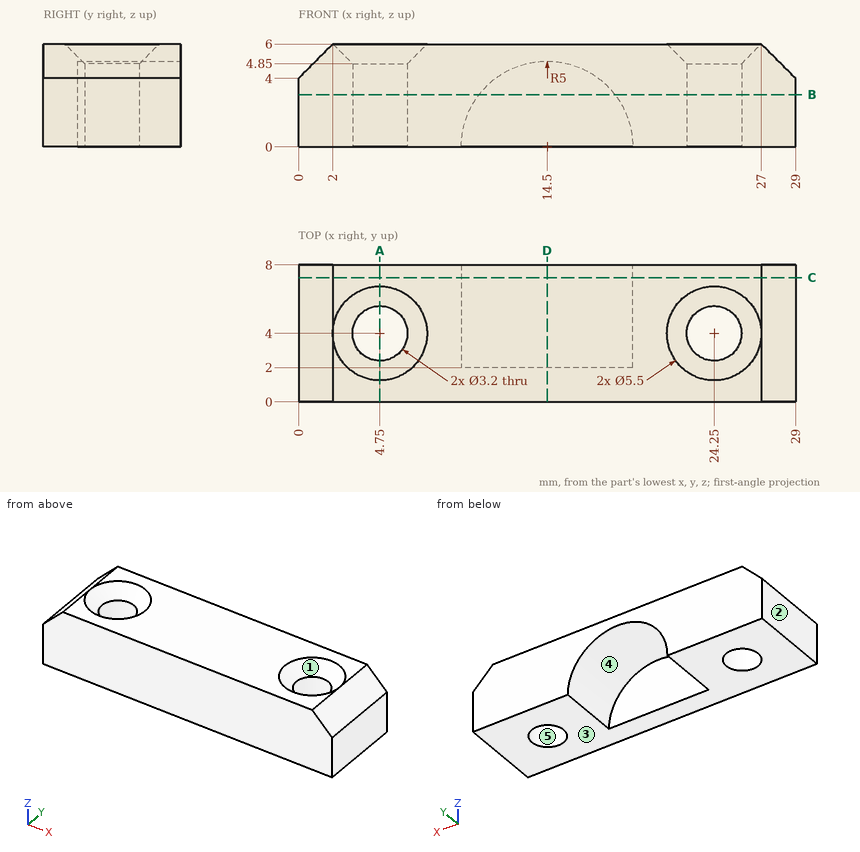
Here's the drawing with two shaded views (mm, measured from the low corner). I have some questions. A direction names the side the tool comes from. Coordinates: 2 decimals unless noted, no trailing zeros. Order: outer loops, then holes, each group sorted by start corner. A loop starts at its lowest first (then second) coordinate and runs counter-clockwise, first axis right, second up.
Item 1: For P1, Ø1.5, axis at x = 16, z = 3, coming from the +Y side; P2, Ø1.5, axis at y = 3, z = 5, coming from the -X side, each with a flat end and sliding along its axis, tell me the tip position at first contact or that it passes through.
Result sheet:
P1: stops at y = 2
P2: stops at x = 0.25
Item 2: If we section it at C-C on y = 7.25: List the corners of the cut face in (x, z) for me.
Result sheet:
outline: (0, 0) - (9.5, 0) arc R5 cw to (19.5, 0) - (29, 0) - (29, 4) - (27, 6) - (2, 6) - (0, 4) - close
Item 3: I need wall thicknesses on line 1 (Y direction, x = 24.25, z = 2.5); line 2 (X direction, y = 3.25, z = 2.9); line 3 (X direction, y = 4.25, z = 5.45). Which ranges of each line are inside material? Lowest first, please.
Result sheet:
line 1: y = 0 to 2.4, 5.6 to 8
line 2: x = 0 to 3.34, 6.16 to 10.43, 18.57 to 22.84, 25.66 to 29
line 3: x = 1.45 to 2.56, 6.94 to 22.06, 26.44 to 27.55
Item 4: For the marked faces 4 and 5, which set-ups out of +Z, -Z, +X, -X, +Y, -Y let a thin tool reach every point of the face, with its end or its side?
Result sheet:
face 4: -Z, +Y
face 5: +Z, -Z
Item 5: If we mould it in two halves opening along X, with no side actions, what happens to the marked faces 1, 2 and 3? For each: +X half, -X half, draft (parallel to the pull), parting line (faces both ways), or undercut.
Result sheet:
face 1: undercut
face 2: -X half
face 3: draft
Item 6: If we section it at B-B on z = 3.05: List the corners of the cut face in (x, y) for me, plus the area to 3 significant figures.
Result sheet:
outline: (0, 0) - (29, 0) - (29, 8) - (18.46, 8) - (18.46, 2) - (10.54, 2) - (10.54, 8) - (0, 8) - close; hole circle Ø3.2 at (4.75, 4); hole circle Ø3.2 at (24.25, 4)
area: 168 mm2
Item 7: If we section it at D-D on x = 14.5: List the corners of the cut face in (y, z) for me, plus the area to 3 significant figures.
Result sheet:
outline: (0, 0) - (2, 0) - (2, 5) - (8, 5) - (8, 6) - (0, 6) - close
area: 18.0 mm2
Item 8: If we section it at A-A on x = 4.75: List the corners of the cut face in (y, z) for me.
Result sheet:
outline: (0, 0) - (2.4, 0) - (2.4, 4.85) - (1.25, 6) - (0, 6) - close; (5.6, 0) - (8, 0) - (8, 6) - (6.75, 6) - (5.6, 4.85) - close
